Geometry: final body of the model. Coordinates: model frame, mm. Face numbers are marked on the shaded views. A direction names the side the tool comes from. Round coordinates to 2 decimals unless told otherwise and drop trailing zeros. Write each loop counter-clockwise with the first axis right and the second up, starting at its lowest first coordinate (ties: lowest second). Pieces come first, ordered by that corner, then holes. Notation, with made-up numbers: M 81,59 L 126,59 A33 ccw 126,94 Z; hole C -4.5,77.5 d8. An arc over 180 degrees is marked long. Use one line per item in the form item = value. Start each with the question number.
from build123d import *

# Parameters (mm, degrees)
F1_DEPTH = 127
F3_DEPTH = 38.1
F4_DEPTH = 273.05
F2_R     = 12.7
F5_DEPTH = 38.1


with BuildPart() as f1:
    # F0 (on Front) → F1 (new body)
    with BuildSketch(Plane.XZ):
        Polygon((31.75, 101.6), (19.05, 101.6), (0, 82.55), (0, 0), (304.8, 0), (304.8, 101.6), (266.7, 101.6), (266.7, 38.1), (31.75, 38.1), align=None)
    extrude(amount=-F1_DEPTH)

    # F2 (on face) → F3 (cut)
    with BuildSketch(Plane.YZ.offset(304.8)):
        with BuildLine():
            Line((0, 101.6), (0, 50.8))
            Line((0, 50.8), (15.875, 50.8))
            Line((15.875, 50.8), (42.406574, 90.350173))
            ThreePointArc((42.406574, 90.350173), (51.547059, 98.611765), (63.5, 101.6))
            Line((63.5, 101.6), (0, 101.6))
        make_face()
        with BuildLine():
            Line((127, 101.6), (63.5, 101.6))
            ThreePointArc((63.5, 101.6), (75.452941, 98.611765), (84.593426, 90.350173))
            Line((84.593426, 90.350173), (111.125, 50.8))
            Line((111.125, 50.8), (127, 50.8))
            Line((127, 50.8), (127, 101.6))
        make_face()
    extrude(amount=-F3_DEPTH, mode=Mode.SUBTRACT)

    # F2 (on face) → F4 (cut)
    with BuildSketch(Plane.YZ.offset(304.8)):
        Polygon((50.8, 16.51), (50.8, 0), (76.2, 0), (76.2, 16.51), (95.25, 16.51), (95.25, 29.21), (76.2, 29.21), (76.2, 38.1), (63.5, 38.1), (50.8, 38.1), (50.8, 29.21), (31.75, 29.21), (31.75, 16.51), align=None)
    extrude(amount=-F4_DEPTH, mode=Mode.SUBTRACT)

    # F2 (on face) → F5 (cut)
    with BuildSketch(Plane.YZ.offset(304.8)):
        with Locations((63.5, 76.2)):
            Circle(F2_R)
    extrude(amount=-F5_DEPTH, mode=Mode.SUBTRACT)


solid = f1.part
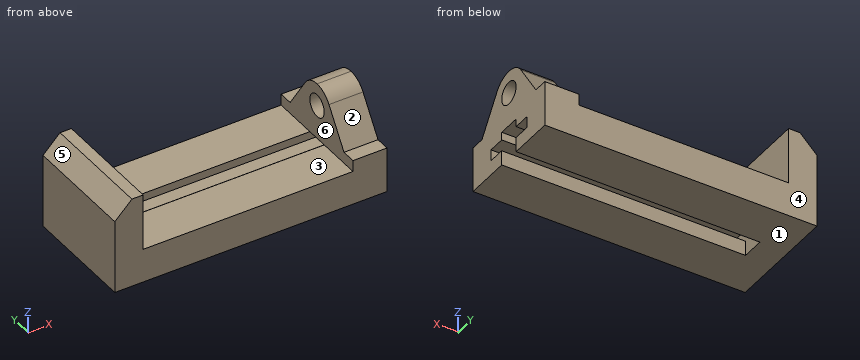
1. Ray query, probe 1 along X at (y, z) = (55.5, 51); probe 2 along Y at (x, z) = (218.5, 24); probe 3 along Z at (x, y) = (78, 24). Return the intervals inside material, ascending.
2. Section query C-C (z = 79.5). Return loops of the section in (x, y).
3. Section query B-B (z = 57.5). Return loops of the section in (x, y).
4. Set-up query: the marked faces 1, 2 and 3. Return all of +Z, -Z, +X, -X, +Y, -Y with unobstructed straight access to the full face (end or side cutting, diameter ignored); none if empty.
5. Contact query for flat-ended pins moving along their axis: pin 1 (21 mm diameter, centred on x = 159, y = 42, fed in from +Z); pin 2 (17.5 mm diameter, centred on x = 290, y = 7, fed in from +Z); pin 3 (4 mm diameter, centred on y = 25.5, z = 81.5, fed in from +X). Output: stop coordinate, or through.
6. Pull-direction query (X, two-part tool) for the marked faces 4, 5 and 6; classes: released by +X, released by -X, zero draft, split by the parting line, or undercut.
7. Section query D-D (y = 36). Return loops of the section in (x, z), then the cut area to 3 significant figures.
8. Section query A-A (x = 261). Return loops of the section in (y, z).
Checks:
q1.probe_1 = 0 to 31.75, 266.7 to 304.8
q1.probe_2 = 0 to 31.75, 95.25 to 127
q1.probe_3 = 0 to 38.1
q2.outline = M 0,0 L 31.75,0 L 31.75,127 L 0,127 Z; M 266.7,35.13 L 304.8,35.13 L 304.8,51.24 L 266.7,51.24 Z; M 266.7,75.76 L 304.8,75.76 L 304.8,91.87 L 266.7,91.87 Z
q3.outline = M 0,0 L 31.75,0 L 31.75,127 L 0,127 Z; M 266.7,20.37 L 304.8,20.37 L 304.8,106.63 L 266.7,106.63 Z
q4.face_1 = -Z, +X, -X, +Y, -Y
q4.face_2 = +Z, +X, -Y
q4.face_3 = +Z, +Y, -Y
q5.pin_1 = 38.1
q5.pin_2 = 50.8
q5.pin_3 = 31.75
q6.face_4 = zero draft
q6.face_5 = released by -X
q6.face_6 = undercut
q7.outline = M 0,0 L 304.8,0 L 304.8,16.51 L 31.75,16.51 L 31.75,29.21 L 304.8,29.21 L 304.8,80.8 L 266.7,80.8 L 266.7,38.1 L 31.75,38.1 L 31.75,101.6 L 19.05,101.6 L 0,82.55 Z
q7.area = 11,600 mm^2
q8.outline = M 0,0 L 50.8,0 L 50.8,16.51 L 31.75,16.51 L 31.75,29.21 L 50.8,29.21 L 50.8,38.1 L 0,38.1 Z; M 76.2,0 L 127,0 L 127,38.1 L 76.2,38.1 L 76.2,29.21 L 95.25,29.21 L 95.25,16.51 L 76.2,16.51 Z
